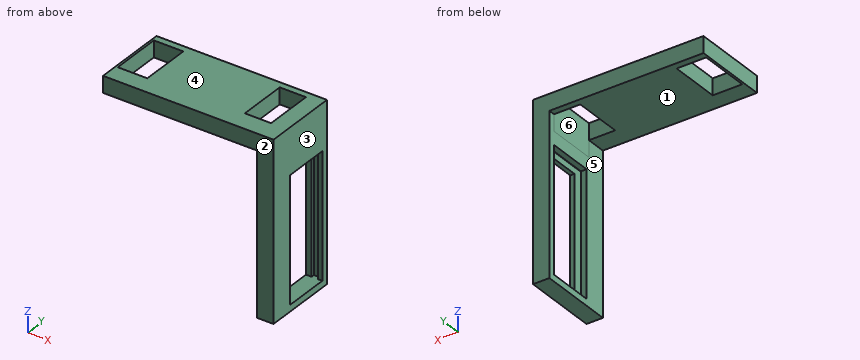
from build123d import *

# Parameters (mm, degrees)
SKETCH040_W                = 15.5
SKETCH040_H                = 9
EXTRUDE038_DEPTH           = 6
EXTRUDE038_PLACEMENT_ANGLE = 90
BOX069_W                   = 8
BOX069_H                   = 15
BOX069_DEPTH               = 15
BOX063_W                   = 2
BOX063_H                   = 14
BOX063_DEPTH               = 37
BOX048_W                   = 2
BOX048_H                   = 19
BOX048_DEPTH               = 40
BOX064_W                   = 8
BOX064_H                   = 14
BOX064_DEPTH               = 38
BOX047_W                   = 5
BOX047_H                   = 23
BOX047_DEPTH               = 49
BOX046_W                   = 52
BOX046_H                   = 23
BOX046_DEPTH               = 5


with BuildPart() as tab001:
    # Sketch040 → Extrude038 (new body)
    with BuildSketch(Plane.XY):
        with Locations((3.19859, 5.867378)):
            Rectangle(SKETCH040_W, SKETCH040_H)
    extrude(amount=EXTRUDE038_DEPTH)


with BuildPart() as tab001_1:
    # Extrude038 placement: moved
    add(tab001.part.moved(Location((142.792, 58.9812, 48.0053))).rotate(Axis((142.792, 58.9812, 48.0053), (0, 0, 1)), EXTRUDE038_PLACEMENT_ANGLE))


with BuildPart() as cables_cut_encoder_piece:
    # Box069 → Box069 (new body)
    with BuildSketch(Plane(origin=(170.769, 55, 44.0053), x_dir=(1, 0, 0), z_dir=(0, 0, 1))):
        with Locations((4, 7.5)):
            Rectangle(BOX069_W, BOX069_H)
    extrude(amount=BOX069_DEPTH)


with BuildPart() as cube016:
    # Box063 → Box063 (new body)
    with BuildSketch(Plane(origin=(201.5, 41, 3), x_dir=(1, 0, 0), z_dir=(0, 0, 1))):
        with Locations((1, 7)):
            Rectangle(BOX063_W, BOX063_H)
    extrude(amount=BOX063_DEPTH)


with BuildPart() as cube010:
    # Box048 → Box048 (new body)
    with BuildSketch(Plane(origin=(203.5, 37, 2), x_dir=(1, 0, 0), z_dir=(0, 0, 1))):
        with Locations((1, 9.5)):
            Rectangle(BOX048_W, BOX048_H)
    extrude(amount=BOX048_DEPTH)


with BuildPart() as encoder_support_slider:
    # Box064 → Box064 (new body)
    with BuildSketch(Plane(origin=(200.5, 41, 2), x_dir=(1, 0, 0), z_dir=(0, 0, 1))):
        with Locations((4, 7)):
            Rectangle(BOX064_W, BOX064_H)
    extrude(amount=BOX064_DEPTH)

    # Fusion125: union Cube016, Cube010
    add(cube016.part)
    add(cube010.part)


with BuildPart() as cube009:
    # Box047 → Box047 (new body)
    with BuildSketch(Plane(origin=(201.768682, 38, 0.005261), x_dir=(1, 0, 0), z_dir=(0, 0, 1))):
        with Locations((2.5, 11.5)):
            Rectangle(BOX047_W, BOX047_H)
    extrude(amount=BOX047_DEPTH)


with BuildPart() as encoder_support_with_tab:
    # Box046 → Box046 (new body)
    with BuildSketch(Plane(origin=(154.768682, 38, 49.005261), x_dir=(1, 0, 0), z_dir=(0, 0, 1))):
        with Locations((26, 11.5)):
            Rectangle(BOX046_W, BOX046_H)
    extrude(amount=BOX046_DEPTH)

    # Fusion094: union Cube009
    add(cube009.part)


with BuildPart() as encoder_support_with_tab_1:
    # Fusion094 placement: moved
    add(encoder_support_with_tab.part.moved(Location((0, -4, 0))))

    # Cut073: cut Encoder support slider
    add(encoder_support_slider.part, mode=Mode.SUBTRACT)


with BuildPart() as encoder_support_with_tab_2:
    # Cut073 placement: moved
    add(encoder_support_with_tab_1.part.moved(Location((-23, 15, 0))))

    # Cut076: cut Cables cut encoder piece
    add(cables_cut_encoder_piece.part, mode=Mode.SUBTRACT)

    # Cut077: cut Tab001
    add(tab001_1.part, mode=Mode.SUBTRACT)


solid = encoder_support_with_tab_2.part
CAD build for the part. Positions are in the model's coordinates, mm. Face numbers are marked on the shaded views. A direction names the side the tool comes from. Give positions to 0.01 mm unless a question says otherwise; leave off trailing zeros. Loops run counter-clockwise (first coordinate to the right, second up) from the corner with the lowest first, then second, coordinate; pieces in that order, holes last. Notation, with made-up numbers: M 74,89 L 107,89 A32 ccw 107,117 Z; hole C -25.5,83 d8. An arc over 180 degrees is marked long. Answer in a Markdown table with one row per item. Add a question column.
Item 1: Band-saw the part on C-C on z = 10. Give the cut face in (x, y).
Item 2: Band-saw the part on B-B on y = 58. Give the number of separate pieces and of enclosed holes in the cut face, then the cut area to 3 significant figures.
Item 3: Drop flat-ended pins along their axis: P1, Ø1, axis at x = 148, y = 62, coming from the -Z side; P2, Ø3, axis at y = 61, z = 44.5, coming from the -X side. Give the stop position or say it passes through.
Item 4: Band-saw the part on A-A on x = 140.5. Give the cut face in (y, z).
Item 5: Tool access for the marked faces 1 and 2: list every direction of +Z, -Z, +X, -X, +Y, -Y with a clear straight run to the whole face (end or side of a thin tool).
Item 6: Probe probe 1 along X at (y, z) = (59.5, 52); probe 2 along Y at (x, z) = (179.5, 6.5); probe 3 along Z at (x, y) = (175, 54.75). List the from-to ranges inside material, lowest first.
Item 7: Band-saw the part on D-D on x = 176. Give the cut face in (y, z), then the cut area to 3 significant figures.
Item 8: Mould opens along X. For the marked faces 3, 4, 5 and 6 say: +X half, -X half, draft (parallel to the pull), parting line (faces both ways), or undercut.
Reply:
| question | item | result |
|---|---|---|
| 1 | outline | M 178.77,49 L 183.77,49 L 183.77,56 L 182.5,56 L 182.5,52 L 180.5,52 L 180.5,56 L 178.77,56 Z; M 178.77,70 L 180.5,70 L 180.5,71 L 182.5,71 L 182.5,70 L 183.77,70 L 183.77,72 L 178.77,72 Z |
| 2 | separate pieces | 4 |
| 2 | enclosed holes | 0 |
| 2 | area | 226 mm^2 |
| 3 | P1 | stops at z = 49.01 |
| 3 | P2 | stops at x = 178.77 |
| 4 | outline | M 49,49.01 L 54.43,49.01 L 54.43,54.01 L 49,54.01 Z; M 69.93,49.01 L 72,49.01 L 72,54.01 L 69.93,54.01 Z |
| 5 | face 1 | -Z, -X, +Y, -Y |
| 5 | face 2 | +Z, -Z, +X, -X, -Y |
| 6 | probe 1 | x = 131.77 to 132.42, 141.42 to 170.77, 178.77 to 183.77 |
| 6 | probe 2 | y = 49 to 56, 70 to 72 |
| 6 | probe 3 | z = 49.01 to 54.01 |
| 7 | outline | M 49,49.01 L 55,49.01 L 55,54.01 L 49,54.01 Z; M 70,49.01 L 72,49.01 L 72,54.01 L 70,54.01 Z |
| 7 | area | 40.0 mm^2 |
| 8 | face 3 | +X half |
| 8 | face 4 | draft |
| 8 | face 5 | -X half |
| 8 | face 6 | undercut |
